```python
from build123d import *

# Parameters (mm, degrees)
SKETCH003_W            = 1.25
SKETCH003_H            = 8.33
PAD003_DEPTH           = 1
BOX019_W               = 27.5
BOX019_H               = 0.8
BOX019_DEPTH           = 1
LINEARPATTERN009_COUNT = 2
LINEARPATTERN009_PITCH = 7
BOX022_W               = 0.8
BOX022_H               = 8
BOX022_DEPTH           = 1
BOX021_W               = 0.8
BOX021_H               = 8
BOX021_DEPTH           = 1
BOX020_W               = 0.65
BOX020_H               = 14
BOX020_DEPTH           = 0.6
LINEARPATTERN011_COUNT = 2
LINEARPATTERN011_PITCH = 12.5
BOX023_W               = 0.65
BOX023_H               = 14
BOX023_DEPTH           = 0.6
LINEARPATTERN010_COUNT = 2
LINEARPATTERN010_PITCH = 13
CYLINDER010_R          = 0.53
CYLINDER010_DEPTH      = 12
CYLINDER009_R          = 2.8
CYLINDER009_DEPTH      = 0.4
BOX025_W               = 1.6
BOX025_H               = 1.8
BOX025_DEPTH           = 1.2
CYLINDER011_R          = 0.6
CYLINDER011_DEPTH      = 2
BOX024_W               = 4
BOX024_H               = 6
BOX024_DEPTH           = 1


with BuildPart() as part:
    # Sketch003 → Pad003 (new body)
    with BuildSketch(Plane.XY):
        with Locations((0.625, 4.165)):
            Rectangle(SKETCH003_W, SKETCH003_H)
    extrude(amount=PAD003_DEPTH)

    # Box019 → Box019 (join)
    with BuildSketch(Plane(origin=(-0.5, 0, 0), x_dir=(1, 0, 0), z_dir=(0, 0, 1))):
        with Locations((13.75, 0.4)):
            Rectangle(BOX019_W, BOX019_H)
    box019 = extrude(amount=BOX019_DEPTH)

    # LinearPattern009: Box019 ×2
    with Locations(*[(0, i * LINEARPATTERN009_PITCH, 0) for i in range(1, LINEARPATTERN009_COUNT)]):
        add(box019)

    # Box022 → Box022 (join)
    with BuildSketch(Plane(origin=(13.2, 0, 0), x_dir=(1, 0, 0), z_dir=(0, 0, 1))):
        with Locations((0.4, 4)):
            Rectangle(BOX022_W, BOX022_H)
    extrude(amount=BOX022_DEPTH)

    # Box021 → Box021 (join)
    with BuildSketch(Plane(origin=(26, 0, 0), x_dir=(1, 0, 0), z_dir=(0, 0, 1))):
        with Locations((0.4, 4)):
            Rectangle(BOX021_W, BOX021_H)
    extrude(amount=BOX021_DEPTH)

    # Box020 → Box020 (join)
    with BuildSketch(Plane(origin=(1, 1, 0.2), x_dir=(0.469472, -0.882948, 0), z_dir=(0, 0, 1))):
        with Locations((0.325, 7)):
            Rectangle(BOX020_W, BOX020_H)
    box020 = extrude(amount=BOX020_DEPTH)

    # LinearPattern011: Box020 ×2
    with Locations(*[(i * LINEARPATTERN011_PITCH, 0, 0) for i in range(1, LINEARPATTERN011_COUNT)]):
        add(box020)

    # Box023 → Box023 (join)
    with BuildSketch(Plane(origin=(13, 0.5, 0.2), x_dir=(0.469472, 0.882948, 0), z_dir=(0, 0, 1))):
        with Locations((0.325, 7)):
            Rectangle(BOX023_W, BOX023_H)
    box023 = extrude(amount=BOX023_DEPTH)

    # LinearPattern010: Box023 ×2
    with Locations(*[(i * LINEARPATTERN010_PITCH, 0, 0) for i in range(1, LINEARPATTERN010_COUNT)]):
        add(box023)

    # Cylinder010 → Cylinder010 (join)
    with BuildSketch(Plane(origin=(0.5, 0, 0.5), x_dir=(1, 0, 0), z_dir=(0, -1, 0))):
        Circle(CYLINDER010_R)
    extrude(amount=CYLINDER010_DEPTH)

    # Cylinder009 → Cylinder009 (join)
    with BuildSketch(Plane(origin=(27, 4.1, 0.6), x_dir=(1, 0, 0), z_dir=(0, 0, 1))):
        Circle(CYLINDER009_R)
    extrude(amount=CYLINDER009_DEPTH)

    # Box025 → Box025 (join)
    with BuildSketch(Plane(origin=(12.8, 7.9, 0), x_dir=(1, 0, 0), z_dir=(0, 0, 1))):
        with Locations((0.8, 0.9)):
            Rectangle(BOX025_W, BOX025_H)
    extrude(amount=BOX025_DEPTH)

    # Cylinder011 → Cylinder011 (cut)
    with BuildSketch(Plane(origin=(13.6, 8.9, 0.5), x_dir=(1, 0, 0), z_dir=(0, 0, 1))):
        Circle(CYLINDER011_R)
    extrude(amount=CYLINDER011_DEPTH, mode=Mode.SUBTRACT)

    # Box024 → Box024 (cut)
    with BuildSketch(Plane(origin=(27, 1, 0), x_dir=(1, 0, 0), z_dir=(0, 0, 1))):
        with Locations((2, 3)):
            Rectangle(BOX024_W, BOX024_H)
    extrude(amount=BOX024_DEPTH, mode=Mode.SUBTRACT)

    # Sphere001 → Sphere001 (revolve)
    with BuildSketch(Plane(origin=(13.55, 9.9, 0.5), x_dir=(1, 0, 0), z_dir=(0, -1, 0))):
        with BuildLine():
            ThreePointArc((0, -0.5), (0.5, 0), (0, 0.5))
            Line((0, 0.5), (0, -0.5))
        make_face()
    revolve(axis=Axis((13.55, 9.9, 0.5), (0, 0, 1)))


with BuildPart() as part_1:
    # Body003 placement: moved
    add(part.part.moved(Location((0, -24, 0))))


solid = part_1.part
```
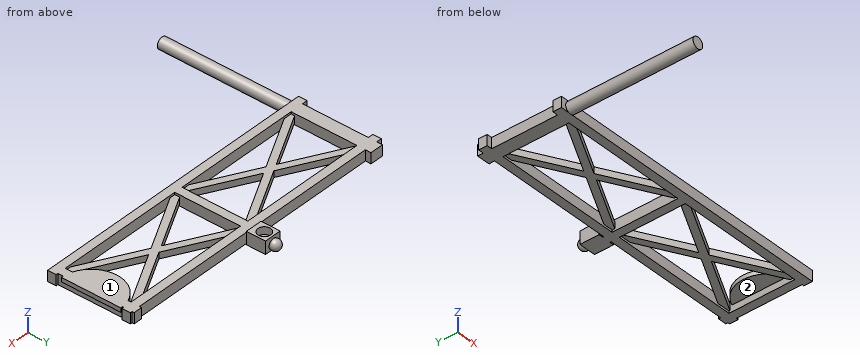
Here's how the part is built. I have some questions about the finished solid (model axes, mm). Face numbers are marked on the shaded views. Round coordinates to 2 decimals unless told otherwise and drop trailing zeros. Order: outer loops, then holes, each group sorted by start corner. A loop starts at its lowest first (then second) coordinate and runs counter-clockwise, first axis right, second up. Notation, with made-up numbers: M 68,72 L 116,72 A24 cw 116,106 Z; hole C -16.5,-9 d6. An arc over 180 degrees is marked long. Answer as CSV lines item,"result".
Item 1: Please list where these lines run through material, in increasing order: L1, parallel to X at y = -15.1, z = 0.75; L2, parallel to Y at x = 13.6, z = 1.05; L3, parallel to Y at x = 3.75, z = 0.95. Write a range as [from, to].
From the geometry:
L1,"[12.8, 13], [14.2, 14.4]"
L2,"[-16.1, -15.7], [-14.5, -14.3]"
L3,"[-24, -23.2], [-17, -16.2]"
Item 2: Imagine slicing it at B-B on x = 5. List the corners of the cut face in (y, z) for me, and give its area (3 significant figures).
From the geometry:
outline,"M -24,0 L -23.2,0 L -23.2,1 L -24,1 Z; M -21.61,0.2 L -20.87,0.2 L -20.87,0.8 L -21.61,0.8 Z; M -19.25,0.2 L -18.51,0.2 L -18.51,0.8 L -19.25,0.8 Z; M -17,0 L -16.2,0 L -16.2,1 L -17,1 Z"
area,"2.48 mm2"
Item 3: Imagine slicing it at C-C on y = -21. Give the number of separate pieces and of enclosed holes in the cut face, and give its area (3 significant figures).
From the geometry:
separate pieces,"7"
enclosed holes,"0"
area,"6.88 mm2"
Item 4: Imagine slicing it at D-D on y = -29. List the corners of the cut face in (x, z) for me, and give its area (3 significant figures).
From the geometry:
outline,"C 0.5,0.5 d1.06"
area,"0.882 mm2"
Item 5: For pin 1 (0.9 mm diameter, centred on x = 25, y = -19, fed in from -Z); pin 2 (5 mm diameter, centred on x = 11.5, y = -20.5, fed in from -Z); pin 3 (0.6 mm diameter, centred on x = 26.5, z = 0.5, fed in from +Y), each with a flat end and sliding along its axis, tell me the tip position at first contact or that it passes through.
From the geometry:
pin 1,"z = 0.6"
pin 2,"z = 0"
pin 3,"y = -16"
Item 6: We'd pull the mould along Y, two halves only. Please class the marked faces 1 and 2: +Y half, -Y half, draft (parallel to the pull), parting line (faces both ways), or undercut.
From the geometry:
face 1,"draft"
face 2,"undercut"
Item 7: Imagine slicing it at A-A on y = -15.1. List the corners of the cut face in (x, z) for me, and give its area (3 significant figures).
From the geometry:
outline,"M 12.8,0 L 14.4,0 L 14.4,1.2 L 14.2,1.2 L 14.2,0.5 L 13,0.5 L 13,1.2 L 12.8,1.2 Z"
area,"1.08 mm2"
